Autodesk Inventor part; units mm, degrees
ref_plane "YZ Plane" through (0, 0, 0) normal (1, 0, 0) x (0, 1, 0)
ref_plane "XZ Plane" through (0, 0, 0) normal (0, 1, 0) x (-1, 0, 0)
ref_plane "XY Plane" through (0, 0, 0) normal (0, 0, 1) x (1, 0, 0)
sketch "Sketch1" plane through (0, 0, 0) normal (0, 0, 1) x (1, 0, 0)
  circle A0 centre (0, 0) radius 2.0955
  circle A1 centre (-12.7, 0) radius 2.0955
  arc A2 (-12.7, 6.35) -> (-12.7, -6.35) centre (-12.7, 0) ccw
  arc A3 (4.9096, 4.0272) -> (0, 6.35) centre (0, 0) ccw
  line L0 (0, 0) -> (32.8335, 0) construction
  line L1 (-12.6049, -6.35) -> (-12.7, -6.35)
  line L2 (-12.7, 6.35) -> (0, 6.35)
  line L3 (1.2503, -27.6905) -> (-9.8373, -7.969)
  arc A4 (-9.8373, -7.969) -> (-12.6049, -6.35) centre (-12.6049, -9.525) ccw
  arc A5 (1.2503, -27.6905) -> (11.8106, -30.8536) centre (8.1692, -23.8006) ccw
  circle A6 centre (8.1692, -23.8006) radius 2.0955
  circle A7 centre (19.454, -17.9745) radius 2.0955
  arc A8 (23.0953, -25.0275) -> (18.7723, -10.0663) centre (19.454, -17.9745) ccw
  line L4 (11.8106, -30.8536) -> (23.0953, -25.0275)
  arc A9 (15.2536, -8.5832) -> (18.7723, -10.0663) centre (18.4204, -5.9855) ccw
  line L5 (15.2536, -8.5832) -> (4.9096, 4.0272)
  point P0 (-10.4687, -6.35)
  dimension "d0" = 4.191
  dimension "d9" = 3.175
  dimension "d10" = 7.9375
  dimension "d11" = 4.191
  dimension "d13" = 4.191
  dimension "d14" = 15.875
  dimension "d15" = 12.7
extrude "Extrusion1" add sketch "Sketch1" along normal blind 1.5875
properties part number "Clamp Gusset" material "Acetal Resin, White"
Geometry: final body of the model. Coordinates: model frame, mm. Give positions to 0.01 mm unless a question says otherwise; leave off trailing zeros. Order: outer loops, then holes, each group sorted by start corner. A loop starts at its lowest first (then second) coordinate and runs counter-clockwise, first axis right, second up. Notation, with made-up numbers: (44.5, 33.5) -> (95.5, 33.5) arc R17 cw to (95.5, 39.5) -> close; hole circle Ø9 at (-8, 21.5). An arc over 180 degrees is marked (long way). Answer as a JSON object with one key per item and string values.
Q1. Draft query along X for faces 1 (the cylindrical face through (7.9, -25.88, 0.78)), 2 (the cylindrical face through (-11.022, -6.773, 0.783)), 3 (the flat face through (10.154, -2.366, 0.783)). Return one class per face: released by +X, released by -X, zero draft, split by the parting line, or undercut.
Entries:
{"face 1": "undercut", "face 2": "released by -X", "face 3": "released by +X"}
Q2. Section B-B (y = 1.5). Output: boundary loops of the cut face in (x, z).
Entries:
{"outline": "(-18.87, 0) -> (-14.16, 0) -> (-14.16, 1.59) -> (-18.87, 1.59) -> close; (-11.24, 0) -> (-1.46, 0) -> (-1.46, 1.59) -> (-11.24, 1.59) -> close; (1.46, 0) -> (6.98, 0) -> (6.98, 1.59) -> (1.46, 1.59) -> close"}
Q3. Material intervals for probe 1 along Y at (x, z) = (-12.7, 0.45); probe 2 along Y at (x, z) = (6.5, 0.25); probe 3 along X at (y, z) = (-9, 0.3), sorted ascending.
Entries:
{"probe 1": "y = -6.35 to -2.1, 2.1 to 6.35", "probe 2": "y = -31.56 to -25.07, -22.53 to 2.09", "probe 3": "x = -9.26 to 15.65"}
Q4. Section D-D (y = -27). Output: boundary loops of the cut face in (x, z), plus the area to 3 significant figures.
Entries:
{"outline": "(0.86, 0) -> (19.27, 0) -> (19.27, 1.59) -> (0.86, 1.59) -> close", "area": "29.2 mm^2"}
Q5. Section C-C (x = 13.5). Output: boundary loops of the cut face in (y, z), plus the area to 3 significant figures.
Entries:
{"outline": "(-29.98, 0) -> (-6.45, 0) -> (-6.45, 1.59) -> (-29.98, 1.59) -> close", "area": "37.4 mm^2"}
Q6. Section A-A (z = 0.6). Output: boundary loops of the cut face in (x, y).
Entries:
{"outline": "(-12.7, -6.35) -> (-12.6, -6.35) arc R3.17 cw to (-9.84, -7.97) -> (1.25, -27.69) arc R7.94 ccw to (11.81, -30.85) -> (23.1, -25.03) arc R7.94 ccw to (18.77, -10.07) arc R4.1 cw to (15.25, -8.58) -> (4.91, 4.03) arc R6.35 ccw to (0, 6.35) -> (-12.7, 6.35) arc R6.35 ccw to start; hole circle Ø4.19 at (-12.7, 0); hole circle Ø4.19 at (0, 0); hole circle Ø4.19 at (8.17, -23.8); hole circle Ø4.19 at (19.45, -17.97)"}
